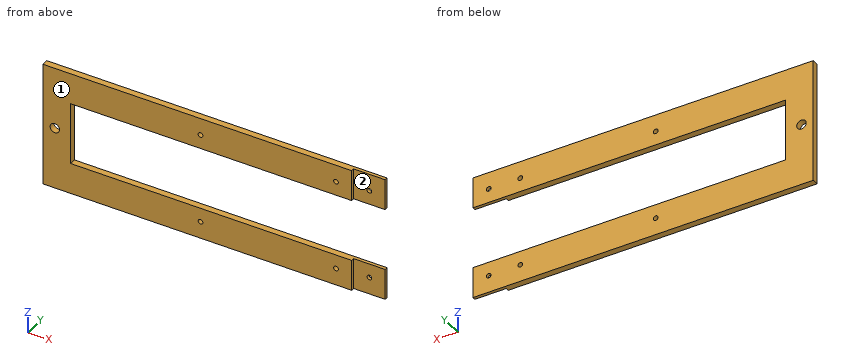
from build123d import *

# Parameters (mm, degrees)
SKETCH1_R           = 1.5
BOSS_EXTRUDE1_DEPTH = 4
SKETCH2_W           = 20
SKETCH2_H           = 2
BOSS_EXTRUDE2_DEPTH = 20
CUT_EXTRUDE1_START  = -10
SKETCH4_R           = 1.5
CUT_EXTRUDE1_DEPTH  = 10


with BuildPart() as part:
    # Sketch1 → Boss-Extrude1 (new body)
    # profile 1 of 2: a face of its own
    with BuildSketch(Plane(origin=(0, 0, 0), x_dir=(1, 0, 0), z_dir=(0, 1, 0))):
        with BuildLine():
            Line((0, 0), (0, -40))
            Line((0, -40), (196, -40))
            Line((196, -40), (196, -20))
            Line((196, -20), (17.5, -20))
            Line((17.5, -20), (17.5, 0))
            Line((17.5, 0), (10.5, 0))
            ThreePointArc((10.5, 0), (7.5, -3), (4.5, 0))
            Line((4.5, 0), (0, 0))
        make_face()
        with Locations(Location((100, -29, 0), (0, 0, 270))):
            Circle(SKETCH1_R, mode=Mode.SUBTRACT)
        with Locations(Location((186, -29, 0), (0, 0, 270))):
            Circle(SKETCH1_R, mode=Mode.SUBTRACT)
    # profile 2 of 2: a face of its own
    with BuildSketch(Plane(origin=(0, 0, 0), x_dir=(1, 0, 0), z_dir=(0, 1, 0))):
        with BuildLine():
            Line((0, 40), (0, 0))
            Line((0, 0), (4.5, 0))
            ThreePointArc((4.5, 0), (7.5, 3), (10.5, 0))
            Line((10.5, 0), (17.5, 0))
            Line((17.5, 0), (17.5, 20))
            Line((17.5, 20), (196, 20))
            Line((196, 20), (196, 40))
            Line((196, 40), (0, 40))
        make_face()
        with Locations(Location((100, 29, 0), (0, 0, 270))):
            Circle(SKETCH1_R, mode=Mode.SUBTRACT)
        with Locations(Location((186, 29, 0), (0, 0, 270))):
            Circle(SKETCH1_R, mode=Mode.SUBTRACT)
    extrude(amount=BOSS_EXTRUDE1_DEPTH)

    # Sketch2 → Boss-Extrude2 (add)
    with BuildSketch(Plane(origin=(196, 0, 0), x_dir=(0, 0, -1), z_dir=(1, 0, 0))):
        with Locations((30, 3)):
            Rectangle(SKETCH2_W, SKETCH2_H)
        with Locations((-30, 3)):
            Rectangle(SKETCH2_W, SKETCH2_H)
    extrude(amount=BOSS_EXTRUDE2_DEPTH)

    # Sketch4 → Cut-Extrude1 (cut)
    with BuildSketch(Plane(origin=(0, 4, 0), x_dir=(1, 0, 0), z_dir=(0, 1, 0)).offset(CUT_EXTRUDE1_START)):
        with Locations(Location((186, 29, 0), (0, 0, 270))):
            Circle(SKETCH4_R)
        with Locations(Location((186, -29, 0), (0, 0, 270))):
            Circle(SKETCH4_R)
        with Locations(Location((206, 29, 0), (0, 0, 270))):
            Circle(SKETCH4_R)
        with Locations(Location((206, -29, 0), (0, 0, 270))):
            Circle(SKETCH4_R)
    extrude(amount=CUT_EXTRUDE1_DEPTH, mode=Mode.SUBTRACT)


solid = part.part
Input: part model. Units: mm. Frame: model coordinates. Face numbers are marked on the shaded views. A direction names the side the tool comes from. Coordinates: 2 decimals unless noted, no trailing zeros. Order: outer loops, then holes, each group sorted by start corner. A loop starts at its lowest first (then second) coordinate and runs counter-clockwise, first axis right, second up.
1. Cut plane A-A, the plane z = 0. Return loops of the section in (x, y).
Checked values:
outline: (0, 0) - (4.5, 0) - (4.5, 4) - (0, 4) - close; (10.5, 0) - (17.5, 0) - (17.5, 4) - (10.5, 4) - close
2. Cut plane C-C, the plane y = 3.4. Return loops of the section in (x, z).
Checked values:
outline: (0, -40) - (216, -40) - (216, -20) - (17.5, -20) - (17.5, 20) - (216, 20) - (216, 40) - (0, 40) - close; hole circle Ø6 at (7.5, 0); hole circle Ø3 at (100, -29); hole circle Ø3 at (100, 29); hole circle Ø3 at (186, -29); hole circle Ø3 at (186, 29); hole circle Ø3 at (206, -29); hole circle Ø3 at (206, 29)
3. Access query for the marked faces 1 and 2. Directions: +Z, -Z, +X, -X, +Y, -Y. A direction counts if a zero-diameter tool reaches every point of the face in a straight line with its end or side. Return the directions, or none.
Checked values:
face 1: +Z, -Z, +X, -X, -Y
face 2: +Z, -Z, +X, -Y
4. Cut plane D-D, the plane z = -35. Return loops of the section in (x, y).
Checked values:
outline: (0, 0) - (196, 0) - (196, 2) - (216, 2) - (216, 4) - (0, 4) - close
5. Contact query for flat-ended pins moving along their axis: P1, Ø16, axis at x = 209.5, z = 26, coming from the -Y side; P2, Ø5, axis at x = 186, z = 29, coming from the -Y side; P3, Ø1.2, axis at y = 1.5, z = -5, coming from the +X side; P4, Ø1.6, axis at y = 0.5, z = 28.5, coming from the +X side. Output: stop coordinate, or through.
Checked values:
P1: stops at y = 2
P2: stops at y = 0
P3: stops at x = 17.5
P4: stops at x = 196
6. Ray query, line 1 along X through (y, z) = (1.55, 29); line 2 along Z through (x, y) = (186, 2.4); line 3 along X through (y, z) = (2.25, 29). Return the intervals inside material, ascending.
Checked values:
line 1: x = 0 to 98.5, 101.5 to 184.5, 187.5 to 196
line 2: z = -40 to -30.5, -27.5 to -20, 20 to 27.5, 30.5 to 40
line 3: x = 0 to 98.5, 101.5 to 184.5, 187.5 to 204.5, 207.5 to 216
7. Cut plane B-B, the plane x = 7.5. Return loops of the section in (y, z).
Checked values:
outline: (0, -40) - (4, -40) - (4, -3) - (0, -3) - close; (0, 3) - (4, 3) - (4, 40) - (0, 40) - close
